Could you check a few things on this model? Use its own coordinates, in mm. Round coordinates to 2 decimals unless told otherwise and drop trailing zeros. Write each loop counter-clockwise with the first axis right and the second up, starting at its lowest first coordinate (ties: lowest second). Pieces come first, ordered by that corner, then holes. Notation, with made-up numbers: (54, 48.25) - (96, 48.25) arc R14 ccw to (96, 63.25) - close; hole circle Ø4 at (88, 57). An arc over 180 degrees is marked (long way). Write each question's results on one line, items separated by ' | '. Start each with the question number.
(1) Imagine slicing it at B-B on z = 18. Write out the boundary of the cut face in (x, y).
(2) Please list where these lines run through material, in increasing order: line 1 (X direction, y = 10, z = 16); line 2 (X direction, y = 36.5, z = -10.5); line 3 (Z direction, x = -214.25, y = 34). Write a range as [from, to].
(3) For P1, Ø3, axis at y = 61.5, z = -12.5, coming from the -X side; P2, Ø1.5, axis at x = -213, y = 43, coming from the +Z side; P3, Ø10, axis at y = 17.5, z = 13, coming from the +X side, each with a flat end and sliding along its axis, tell me the tip position at first contact or that it passes through.
(4) Imagine slicing it at C-C on z = -7.5. Write out the boundary of the cut face in (x, y), then the cut area to 3 significant figures.
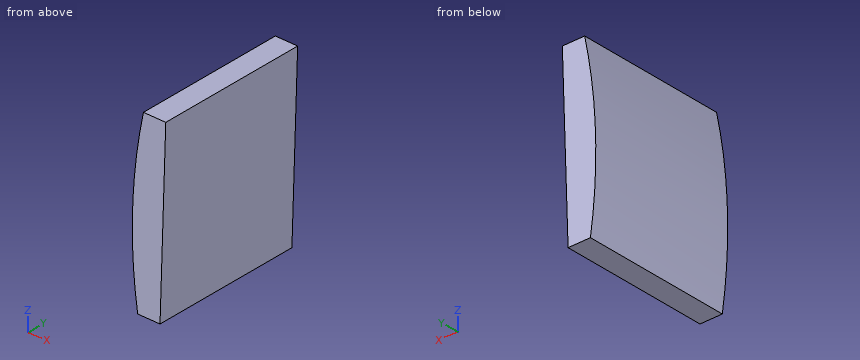
Autodesk Inventor part; units mm, degrees
ref_plane "Work Plane1" through (-224.8836, 0, 7.236) normal (0.9994827, 0, -0.03216) x (0, 1, 0)
ref_plane "YZ Plane" through (0, 0, 0) normal (1, 0, 0) x (0, 1, 0)
ref_plane "XZ Plane" through (0, 0, 0) normal (0, 1, 0) x (-1, 0, 0)
sketch "Sketch1" plane through (0, 0, 0) normal (0, 1, 0) x (-1, 0, 0)
  point P0 (0, 0)
sketch "Sketch2" plane through (0, 0, 0) normal (0, 1, 0) x (-1, 0, 0)
  circle A0 centre (0, 0) radius 225
  dimension "d0" = 450
extrude "Extrusion1" add sketch "Sketch2" along normal blind 70
sketch "Sketch3" plane through (0, 70, 0) normal (0, 1, 0) x (1, 0, 0)
  circle A0 centre (0, 0) radius 225
  line L0 (-222.5878, 32.8586) -> (-220.015, -47.1001)
  dimension "d3" = 80
split body "Split1" sketch "Sketch3" result one side removed curves L0 removed pieces at (-39.9451, 0.5, -49.4831)
sketch "Sketch4" plane through (-220.015, 0, 47.1001) normal (0.9994827, 0, -0.03216) x (-0.03216, 0, -0.9994827)
  line L0 (80, 70) -> (0, 70)
  line L1 (0, 70) -> (80, 70)
  line L2 (80, 70) -> (80, 0)
  line L3 (80, 0) -> (0, 0)
  line L4 (0, 0) -> (0, 70)
  point P0 (40, 0)
extrude "Extrusion2" add sketch "Sketch4" along normal blind 10
sketch "Sketch5" plane through (-210.0201, 0, 46.7785) normal (0.9994827, 0, -0.03216) x (-0.03216, 0, -0.9994827)
  point P0 (40, 0)
ref_plane "Work Plane1" through (-224.8836, 0, 7.236) normal (0.9994827, 0, -0.03216) x (0, 1, 0)
properties part number "Speaker Mount 1"
Response:
1) outline: (-224.28, 0) - (-210.95, 0) - (-210.95, 70) - (-224.28, 70) - close
2) line 1: [-224.43, -211.01] | line 2: [-224.75, -211.86] | line 3: [-33.13, 46.91]
3) P1: x = -224.73 | P2: z = 46.9 | P3: x = -210.95
4) outline: (-224.87, 0) - (-211.77, 0) - (-211.77, 70) - (-224.87, 70) - close | area: 918 mm²
